```python
from build123d import *

# Parameters (mm, degrees)
F1_DEPTH = 3
F3_D     = 6.6


with BuildPart() as f1:
    # F0 (on Front) → F1 (new body)
    with BuildSketch(Plane.XZ):
        Polygon((-236.2583571076, 137.1082649553), (-236.2583571076, -523.2917350447), (271.7416428924, -523.2917350447), (271.7416428924, 137.1082649553), (220.9416428924, 238.7082649553), (-185.4583571076, 238.7082649553), align=None)
        with BuildLine():
            ThreePointArc((-185.4583571076, 111.7082649553), (-170.5793815919, 147.6292894396), (-134.6583571076, 162.5082649553))
            Line((-134.6583571076, 162.5082649553), (170.1416428924, 162.5082649553))
            ThreePointArc((170.1416428924, 162.5082649553), (206.0626673766, 147.6292894396), (220.9416428924, 111.7082649553))
            Line((220.9416428924, 111.7082649553), (220.9416428924, -66.0917350447))
            ThreePointArc((220.9416428924, -66.0917350447), (206.0626673766, -102.012759529), (170.1416428924, -116.8917350447))
            Line((170.1416428924, -116.8917350447), (-134.6583571076, -116.8917350447))
            ThreePointArc((-134.6583571076, -116.8917350447), (-170.5793815919, -102.012759529), (-185.4583571076, -66.0917350447))
            Line((-185.4583571076, -66.0917350447), (-185.4583571076, 111.7082649553))
        make_face(mode=Mode.SUBTRACT)
    extrude(amount=F1_DEPTH)

    # F3 (through all)
    with Locations(Plane.XZ.offset(3)):
        with Locations((-223.7583571076, -497.8917350447), (-223.7583571076, -345.4917350447), (-223.7583571076, -193.0917350447), (-223.7583571076, -40.6917350447), (-223.7583571076, 111.7082649553), (-160.0583571076, 226.2082649553), (17.7416428924, 226.2082649553), (195.5416428924, 226.2082649553), (259.2416428924, 111.7082649553), (259.2416428924, -40.6917350447), (259.2416428924, -193.0917350447), (259.2416428924, -345.4917350447), (259.2416428924, -497.8917350447)):
            Hole(F3_D / 2)


solid = f1.part
```
Check sheet for the modelled part. Datum: model origin and axes. Units: mm. A direction names the side the tool comes from. Coordinates: 2 decimals unless noted, no trailing zeros. Write each loop counter-clockwise with the first axis right and the second up, starting at its lowest first coordinate (ties: lowest second). Pieces come first, ordered by that corner, then holes. Notation, with made-up numbers: M -15.75,62 L 9.25,62 A14 cw 9.25,79 Z; hole C 31.5,27 d3. An arc over 180 degrees is marked long. Use one line per item in the form item = value.
Item 1: Sectioned sample at B-B, the plane x = 78. Record the cut outline in (y, z).
Answer below:
outline = M -3,-523.29 L 0,-523.29 L 0,-116.89 L -3,-116.89 Z; M -3,162.51 L 0,162.51 L 0,238.71 L -3,238.71 Z
Item 2: Set-up check for faces 5 (the face through (-170.972, -1.479, 147.232)), 6 (the face through (14, 0, -222)): record each of +Z, -Z, +X, -X, +Y, -Y from which the full face is reachable in a straight line by a thin tool's end or side.
Answer below:
face_5 = +Y, -Y
face_6 = +Z, -Z, +X, -X, +Y
Item 3: Sectioned sample at C-C, the plane y = -2.55. State how many separate pieces and enclosed holes the cut face has, and give its area (3 significant figures).
Answer below:
separate_pieces = 1
enclosed_holes = 14
area = 270,000 mm^2
Item 4: Sectioned sample at A-A, the plane z = 68.5. Record the cut outline in (x, y), and give its area (3 significant figures).
Answer below:
outline = M -236.26,-3 L -185.46,-3 L -185.46,0 L -236.26,0 Z; M 220.94,-3 L 271.74,-3 L 271.74,0 L 220.94,0 Z
area = 305 mm^2
Item 5: Material ranges on L1, parallel to X at y = -2.15, z = 64; L2, parallel to Z at x = -66, y = -1.45; L3, parallel to X at y = -2.3, z = -345, recorded low to high. Write a range as from..to.
Answer below:
L1 = -236.26..-185.46, 220.94..271.74
L2 = -523.29..-116.89, 162.51..238.71
L3 = -236.26..-227.02, -220.5..255.98, 262.5..271.74
Item 6: Sectioned sample at D-D, the plane x = 231.5. Record the cut outline in (y, z), and give its area (3 significant figures).
Answer below:
outline = M -3,-523.29 L 0,-523.29 L 0,217.59 L -3,217.59 Z
area = 2,220 mm^2
Item 7: Release check for a two-part mould opening along X. For faces 1 (the face through (-170.18, -1.48, -102.41)), 2 (the face through (-210.503, -1.479, 188.619)), 3 (the face through (246.697, -1.479, 187.197)), 4 (the face through (14, -3, -222)) record: pulls with the +X half, pulls with the -X half, needs draft (parallel to the pull), parting line crosses it, or undercut.
Answer below:
face_1 = undercut
face_2 = pulls with the -X half
face_3 = pulls with the +X half
face_4 = needs draft
